Read the model definition and answer for the solid it produces. Units are mm, in the model's axes. Face numbers are marked on the shaded views. A direction names the side the tool comes from. Coordinates: 2 decimals unless noted, no trailing zeros. Order: outer loops, then holes, each group sorted by start corner. A loop starts at its lowest first (then second) coordinate and runs counter-clockwise, first axis right, second up. Notation, with made-up numbers: M -32.5,-14.75 L 2.5,-14.75 A32 ccw 2.5,14.25 Z; hole C 86.25,61 d10. An arc over 180 degrees is marked long. Use a Markdown table: item, result. Add a question column.
1) Find the intervals of material crossed by probe 1 along Y at (x, z) = (36.5, 9.75); probe 2 along Y at (x, z) = (40, 6.5); probe 3 along Y at (x, z) = (-19, 6), in increasing order. Write a range as [from, to].
2) Find section D-D on x = -41. Write down the section's boundary in (y, z), plus the area to 3 significant figures.
3) Each of these flat-tipped pins is pushed along its axis until it touches: pin 1 Ø4 at (y, z) = (20, 11) entering from -X; pin 2 Ø6 at (x, z) = (-4, 2) entering from -Y; pin 3 Ø4 at (y, z) = (36, 8) entering from -X. Where does it stop, or does it pass through?
4) Find section B-B on z = 8.5. Write down the section's boundary in (x, y), plus the area to 3 significant figures.
5) The mould has two halves that part along X. Classify the marked faces 4, 5, 6 and 7: released by +X, released by -X, zero draft, split by the parting line, or undercut.
6) Find section C-C on x = 6.5. Write down the section's boundary in (y, z), plus the area to 3 significant figures.
7) For the marked faces 1, 2 and 3, determine the directions among +Z, -Z, +X, -X, +Y, -Y from which every point of the face is accessible in a straight line to the end or side of a thin tool.
8) Find section A-A on y = 35.5. Write down the section's boundary in (x, z), plus the area to 3 significant figures.
from build123d import *

# Parameters (mm, degrees)
F0_R     = 50.8
F1_DEPTH = 12.7
F3_DEPTH = 25.4
F4_T     = -1.27
F5_R     = 7.5301536969
F5_R_2   = 14.5632315152
F5_R_3   = 12.2458947517
F5_R_4   = 13.1514676022
F6_DEPTH = 25.4


with BuildPart() as f1:
    # F0 (on Top) → F1 (new body)
    with BuildSketch(Plane.XY):
        Circle(F0_R)
    extrude(amount=F1_DEPTH)

    # F2 (on face) → F3 (cut)
    with BuildSketch(Plane.XY.offset(12.7)):
        with BuildLine():
            Line((42.7394116495, 27.4587452709), (0, 0))
            Line((0, 0), (48.1856271225, -16.0868063582))
            ThreePointArc((48.1856271225, -16.0868063582), (50.1421472308, -8.1489306714), (50.8, 0))
            ThreePointArc((50.8, 0), (48.7432154858, 14.3087016917), (42.7394116495, 27.4587452709))
        make_face()
    extrude(amount=-F3_DEPTH, mode=Mode.SUBTRACT)

    # F4
    f4_openings = [f1.faces().sort_by_distance(p)[0] for p in [
        (-5.386062, -0.673631, 12.7),
    ]]
    offset(amount=F4_T, openings=f4_openings, kind=Kind.INTERSECTION)

    # F5 (on face) → F6 (cut)
    with BuildSketch(Plane(origin=(0, 0, 0), x_dir=(1, 0, 0), z_dir=(0, 0, -1))):
        with Locations((-19.0832894295, 30.751734972)):
            Circle(F5_R)
        with Locations((10.1048983634, 25.5627222359)):
            Circle(F5_R_2)
        with Locations((-3.0838376842, -33.6784869432)):
            Circle(F5_R_3)
        with Locations((-32.4882343411, 4.3742610142)):
            Circle(F5_R_4)
    extrude(amount=-F6_DEPTH, mode=Mode.SUBTRACT)


solid = f1.part
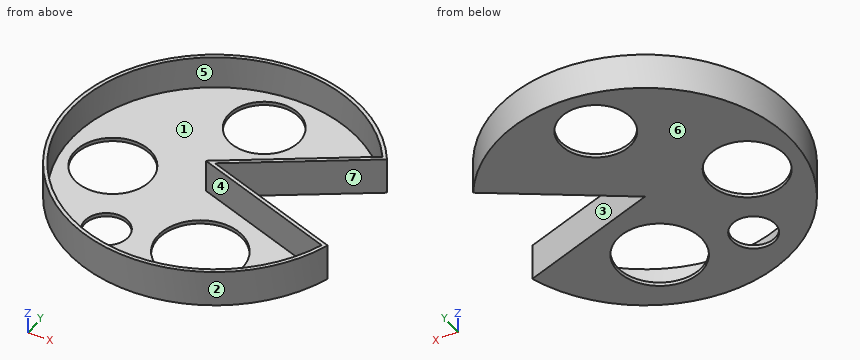
Check result:
| question | item | result |
|---|---|---|
| 1 | probe 1 | y = [-35.33, -33.48], [-13.52, -12.19], [23.45, 24.96], [33.48, 35.33] |
| 1 | probe 2 | y = [-31.32, -29.21], [-14.69, -13.35], [25.7, 27.21], [29.21, 31.32] |
| 1 | probe 3 | y = [-47.11, -45.74], [45.74, 47.11] |
| 2 | outline | M -29.99,0 L -14.4,0 L -14.4,1.27 L -27.79,1.27 L -27.79,12.7 L -29.99,12.7 Z; M 5.65,0 L 29.99,0 L 29.99,12.7 L 27.79,12.7 L 27.79,1.27 L 5.65,1.27 Z |
| 2 | area | 101 mm2 |
| 3 | pin 1 | stops at x = -47.5 |
| 3 | pin 2 | stops at y = -50.79 |
| 3 | pin 3 | stops at x = -37.74 |
| 4 | outline | M 0,0 L 42.74,27.46 A50.8 ccw long 48.19,-16.09 Z; hole M -2.92,-0.36 L 40.97,27.83 A49.53 ccw long 46.56,-16.88 Z |
| 4 | area | 473 mm2 |
| 5 | face 4 | undercut |
| 5 | face 5 | undercut |
| 5 | face 6 | zero draft |
| 5 | face 7 | released by +X |
| 6 | outline | M -50.38,0 L -39.67,0 L -39.67,1.27 L -49.1,1.27 L -49.1,12.7 L -50.38,12.7 Z; M -11.45,0 L -2.17,0 L -2.17,12.7 L -3.51,12.7 L -3.51,1.27 L -11.45,1.27 Z; M 4.18,0 L 26.06,0 L 26.06,1.27 L 5.69,1.27 L 5.69,12.7 L 4.18,12.7 Z; M 41.3,0 L 50.38,0 L 50.38,12.7 L 49.1,12.7 L 49.1,1.27 L 41.3,1.27 Z |
| 6 | area | 127 mm2 |
| 7 | face 1 | +Z |
| 7 | face 2 | +Z, -Z |
| 7 | face 3 | +Z, -Z, +X |
| 8 | outline | M -36.34,0 L -15.19,0 L -15.19,1.27 L -34.54,1.27 L -34.54,12.7 L -36.34,12.7 Z; M 9.03,0 L 36.34,0 L 36.34,12.7 L 34.54,12.7 L 34.54,1.27 L 9.03,1.27 Z |
| 8 | area | 103 mm2 |
